from build123d import *

# Parameters (mm, degrees)
F0_W     = 23.2594013214
F0_H     = 54.8999868333
F0_R     = 16.9272487263
F1_DEPTH = 6


# Not quite as in the source:
# - a feature names something its author has since deleted; it is built from what else it names


with BuildPart() as f1:
    # F0 (on Front) → F1 (new body)
    with BuildSketch(Plane.XZ):
        with BuildLine():
            add(Edge.make_bspline(
                [(266.3061527885, -172.8736048774), (266.4418306907, -161.1180388855), (266.4673413702, -154.0153294904), (266.4976486654, -153.6832076827)],
                knots=[239.4581463651, 239.4581463651, 239.4581463651, 239.4581463651, 284.4819853699, 284.4819853699, 284.4819853699, 284.4819853699], degree=3))
            Line((266.4976486654, -153.6832076827), (232.4976486654, -153.6832076827))
            Line((232.4976486654, -153.6832076827), (232.4976486654, -158.6832076827))
            Line((232.4976486654, -158.6832076827), (198.4976486654, -158.6832076827))
            Line((198.4976486654, -158.6832076827), (198.4976486654, -416.6832076827))
            Line((198.4976486654, -416.6832076827), (208.4976486654, -416.6832076827))
            Line((208.4976486654, -416.6832076827), (208.4976486654, -436.6832076827))
            Line((208.4976486654, -436.6832076827), (237.4976486654, -436.6832076827))
            add(Edge.make_bspline(
                [(237.4976486654, -436.6832076827), (261.7467447475, -429.5284690744), (265.5845533054, -235.3952845947), (266.3061527885, -172.8736048774)],
                knots=[0, 0, 0, 0, 239.4581463651, 239.4581463651, 239.4581463651, 239.4581463651], degree=3))
        make_face()
        with Locations((221.1196951035, -377.0302243151)):
            Rectangle(F0_W, F0_H, mode=Mode.SUBTRACT)
        with Locations((228.8340181112, -220.9526370094)):
            Circle(F0_R, mode=Mode.SUBTRACT)
        with BuildLine():
            add(Edge.make_bspline(
                [(237.4976486654, 129.3167923173), (261.7467447475, 122.1620537089), (265.5845533054, -71.9711307708), (266.3061527885, -134.492810488)],
                knots=[0, 0, 0, 0, 239.4581463651, 239.4581463651, 239.4581463651, 239.4581463651], degree=3))
            Line((237.4976486654, 129.3167923173), (208.4976486654, 129.3167923173))
            Line((208.4976486654, 129.3167923173), (208.4976486654, 109.3167923173))
            Line((208.4976486654, 109.3167923173), (198.4976486654, 109.3167923173))
            Line((198.4976486654, 109.3167923173), (198.4976486654, -148.6832076827))
            Line((198.4976486654, -148.6832076827), (232.4976486654, -148.6832076827))
            Line((232.4976486654, -148.6832076827), (232.4976486654, -153.6832076827))
            Line((232.4976486654, -153.6832076827), (266.4976486654, -153.6832076827))
            add(Edge.make_bspline(
                [(266.3061527885, -134.492810488), (266.4418306907, -146.24837648), (266.4673413702, -153.3510858751), (266.4976486654, -153.6832076827)],
                knots=[239.4581463651, 239.4581463651, 239.4581463651, 239.4581463651, 284.4819853699, 284.4819853699, 284.4819853699, 284.4819853699], degree=3))
        make_face()
        with Locations((228.8340181112, -86.4137783561)):
            Circle(F0_R, mode=Mode.SUBTRACT)
        with Locations((221.1196951035, 69.6638089497)):
            Rectangle(F0_W, F0_H, mode=Mode.SUBTRACT)
    extrude(amount=F1_DEPTH)


solid = f1.part
The model under review builds one solid part; all positions refer to its coordinate system, in mm. Round coordinates to 2 decimals unless told otherwise and drop trailing zeros. Write each loop counter-clockwise with the first axis right and the second up, starting at its lowest first coordinate (ties: lowest second). Pieces come first, ordered by that corner, then holes. Notation, with made-up numbers: M 23,63.5 L 30,63.5 A11 cw 30,69.5 Z; hole C 78.5,-8.5 d1. An arc over 180 degrees is marked long. Use a Markdown table: item, result. Add a question column.
Q1. To check wall thickness, follow line 1 (Z direction, x = 241, y = -1.5); line 2 (Z direction, x = 232, y = -4); line 3 (Z direction, x = 216.5, y = -4). State the ranges of each line that lie inside material, in increasing order.
Q2. The part is to be moulded in two halves that separate along Z. For faces 1 (the face through (240, 0, -150)), 2 (the face through (216.36, -2.96, -209.51)), say which applies: pulls with the +Z half, pulls with the -Z half, needs draft (parallel to the pull), parting line crosses it, or undercut.
Q3. We need section B-B, the plane y = -3. Count the separate pieces of the cut face and the enclosed holes in it, plus the area to 3 significant figures.
Q4. We need section A-A, the plane x = 216.5. State the section outline as (y, z) points, plus the area to 3 significant figures.
Q5. Insertion check: pin 1 (3 mm diameter, centred on x = 203, y = -3.5, fed in from +Z); pin 2 (3 mm diameter, centred on y = -4, z = -429, fed in from -X); pin 3 (12 mm diameter, centred on x = 255.5, z = -297, fed in from +Y). Each pin has a flat end and moves straight along its axis. Give the tip position at first contact, or say it passes through.
Findings below:
| question | item | result |
|---|---|---|
| 1 | line 1 | z = -434.23 to -232.72, -209.18 to -98.18, -74.64 to 126.86 |
| 1 | line 2 | z = -436.68 to -404.48, -349.58 to -237.58, -204.32 to -158.68, -148.68 to -103.04, -69.79 to 42.21, 97.11 to 129.32 |
| 1 | line 3 | z = -436.68 to -404.48, -349.58 to -232.55, -209.36 to -158.68, -148.68 to -98.01, -74.82 to 42.21, 97.11 to 129.32 |
| 2 | face 1 | needs draft |
| 2 | face 2 | undercut |
| 3 | separate pieces | 1 |
| 3 | enclosed holes | 4 |
| 3 | area | 29,900 mm² |
| 4 | outline | M -6,-436.68 L 0,-436.68 L 0,-404.48 L -6,-404.48 Z; M -6,-349.58 L 0,-349.58 L 0,-232.55 L -6,-232.55 Z; M -6,-209.36 L 0,-209.36 L 0,-158.68 L -6,-158.68 Z; M -6,-148.68 L 0,-148.68 L 0,-98.01 L -6,-98.01 Z; M -6,-74.82 L 0,-74.82 L 0,42.21 L -6,42.21 Z; M -6,97.11 L 0,97.11 L 0,129.32 L -6,129.32 Z |
| 4 | area | 2,400 mm² |
| 5 | pin 1 | stops at z = 109.32 |
| 5 | pin 2 | stops at x = 208.5 |
| 5 | pin 3 | stops at y = 0 |
